from build123d import *

# Parameters (mm, degrees)
F0_W     = 42
F0_H     = 80
F0_R     = 16
F1_DEPTH = 225
F2_R     = 16
F2_R_2   = 14
F3_DEPTH = 100
F4_R     = 2.5
F5_DEPTH = 25
F6_R     = 2.5
F7_DEPTH = 25
F8_SIZE  = 1


with BuildPart() as f1:
    # F0 (on Front) → F1 (new body)
    with BuildSketch(Plane.XZ):
        Rectangle(F0_W, F0_H)
        with Locations((0, -19)):
            Circle(F0_R, mode=Mode.SUBTRACT)
    extrude(amount=-F1_DEPTH)

    # F2 (on face) → F3 (cut)
    with BuildSketch(Plane(origin=(-21, 0, 0), x_dir=(0, -1, 0), z_dir=(-1, 0, 0))):
        with Locations((-204, 19)):
            Circle(F2_R)
        with Locations((-56, 19)):
            Circle(F2_R_2)
        with Locations((-21, 19)):
            Circle(F2_R)
    extrude(amount=-F3_DEPTH, mode=Mode.SUBTRACT)

    # F4 (on face) → F5 (cut)
    with BuildSketch(Plane.XY.offset(40)):
        with Locations((0, 21)):
            Circle(F4_R)
        with Locations((0, 56)):
            Circle(F4_R)
        with Locations((0, 204)):
            Circle(F4_R)
    extrude(amount=-F5_DEPTH, mode=Mode.SUBTRACT)

    # F6 (on face) → F7 (cut)
    with BuildSketch(Plane(origin=(0, 0, -40), x_dir=(1, 0, 0), z_dir=(0, 0, -1))):
        with Locations((0, -21)):
            Circle(F6_R)
        with Locations((0, -204)):
            Circle(F6_R)
        with Locations((0, -105)):
            Circle(F6_R)
        with Locations((0, -155)):
            Circle(F6_R)
    extrude(amount=-F7_DEPTH, mode=Mode.SUBTRACT)

    # F8
    f8_edges = [f1.edges().sort_by_distance(p)[0] for p in [
        (-21, 70, 19),
        (-21, 37, 19),
        (-16, 0, -19),
        (-21, 220, 19),
        (21, 37, 19),
        (21, 70, 19),
        (21, 220, 19),
        (-16, 225, -19),
    ]]
    chamfer(f8_edges, length=F8_SIZE)


solid = f1.part
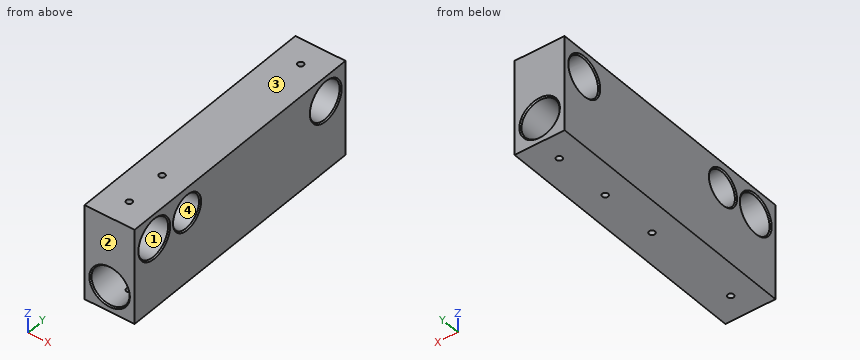
Design review of the part built by this model. Coordinates are the model's own, in mm. Face numbers are marked on the shaded views. Round coordinates to 2 decimals unless told otherwise and drop trailing zeros. Loops run counter-clockwise (first coordinate to the right, second up) from the corner with the lowest first, then second, coordinate; pieces in that order, holes last. Notation, with made-up numbers: M 1,81.25 L 34,81.25 A21 ccw 34,108.25 Z; hole C -23,-39 d6. An arc over 180 degrees is marked long. Answer as a JSON object with one key per item and string values.
Item 1: Wall thickness on L1, parallel to Y at x = 0, z = -36.5; L2, parallel to X at y = 204, z = 37; L3, parallel to Z at x = -7, y = 204: over which ranges is each line inside the solid? List them lowest first. Write a range as from..to.
Answer sheet:
{"L1": "y = 0..18.5, 23.5..102.5, 107.5..152.5, 157.5..201.5, 206.5..225", "L2": "x = -21..-2.5, 2.5..21", "L3": "z = -40..-33.39, -4.61..3, 35..40"}
Item 2: We need section A-A on z = -19. Give the boundary of the cut face in (x, y), and give its area (3 significant figures).
Answer sheet:
{"outline": "M -21,0 L -17,0 L -16,1 L -16,224 L -17,225 L -21,225 Z; M 16,1 L 17,0 L 21,0 L 21,225 L 17,225 L 16,224 Z", "area": "2,250 mm^2"}
Item 3: We need section C-C on y = 96. Give the boundary of the cut face in (x, z), and give its area (3 significant figures).
Answer sheet:
{"outline": "M -21,-40 L 21,-40 L 21,40 L -21,40 Z; hole C 0,-19 d32", "area": "2,560 mm^2"}
Item 4: We need section B-B on x = 0. State how many separate pieces and enclosed holes the cut face has, and give its area (3 significant figures).
Answer sheet:
{"separate pieces": "6", "enclosed holes": "0", "area": "8,390 mm^2"}
Item 5: The part is to be moulded in two halves that separate along Z. For the marked faces 1, 2, 3 and 4, say which applies: pulls with the +Z half, pulls with the -Z half, needs draft (parallel to the pull), parting line crosses it, or undercut.
Answer sheet:
{"face 1": "undercut", "face 2": "needs draft", "face 3": "pulls with the +Z half", "face 4": "undercut"}
Item 6: Clearance check with flat-ended pins moving along their axes: P1, Ø4, axis at x = 0, y = 21, coming from the +Z side; P2, Ø2, axis at x = -14, z = -26, coming from the +Y side; P3, Ø10, axis at x = 9.5, z = -19.5, coming from the -Y side; P4, Ø4, axis at x = 0, y = 204, coming from the -Z side. State where each tip first meets the part, or that it passes through.
Answer sheet:
{"P1": "stops at z = 3.13", "P2": "stops at y = 224.65", "P3": "passes through", "P4": "stops at z = -3.13"}
